Can you work these out from the model? Positions are in its coordinate system, mm. Face numbers are marked on the shaded views. A direction names the side the tool comes from. Round coordinates to 2 decimals unless told otherwise and drop trailing zeros. Order: outer loops, then holes, each group sorted by start corner. A loop starts at its lowest first (then second) coordinate and runs counter-clockwise, first axis right, second up. Notation, with made-up numbers: (10.25, -12) -> (64.25, -12) arc R29 ccw to (64.25, 13) -> close; hole circle Ø3 at (10.5, 52.25). An arc over 180 degrees is marked (long way). Use a Markdown table: item, result. Add a question column.
Q1. If we section it at A-A on y = 0: List the corners of the cut face in (x, z) for me, plus the area to 3 significant figures.
Q2. If we section it at D-D on z = 18.5: List the corners of the cut face in (x, y) for me, plus the area to 3 significant figures.
Q3. I'm going to push flat-ended pins straight in: pin 1 Ø3 at (x, y) = (25.5, -107) entering from -Z; pin 2 Ø2 at (x, z) = (23.5, 11) entering from +Y; pin 3 Ø6 at (x, y) = (16, 12) entering from +Z. Where does each tip first touch, or does it pass through?
Q4. If we section it at B-B on z = 0: List the corners of the cut face in (x, y) for me.
Q5. For the marked faces 1, 2 and 3, which set-ups out of +Z, -Z, +X, -X, +Y, -Y let a thin tool reach every point of the face, with its end or its side?
Q6. If we section it at C-C on y = -104.5: List the corners of the cut face in (x, z) for me.
Q7. I need wall thicknesses on line 1 along Y through (x, z) = (13, 43.5); line 2 along Y through (x, z) = (15.75, 35.5); line 3 along Z through (x, y) = (4.25, 44). Which ranges of each line are inside material? Lowest first, please. Write a range as [from, to].
Q8. We'd pull the mould along Y, two halves only. Please class the marked faces 4, 5, 6 and 7: +Y half, -Y half, draft (parallel to the pull), parting line (faces both ways), or undercut.
```python
from build123d import *

# Parameters (mm, degrees)
BASPROSKE_W              = 30
BASPROSKE_H              = 55
TOOTHCUT_DEPTH           = 84.366660003
TEETHCUTS_COUNT          = 20
BORSKE_R                 = 2.5
BORE_DEPTH               = 50.0000508
EXTRUDE_1_DEPTH          = 30
CUT_EXTRUDE_1_DEPTH      = 158.555338193
CUT_EXTRUDE_1_DEPTH_BACK = 158.555338193
SKETCH_7_R               = 2.5


with BuildPart() as part:
    # BasProSke → Base-Revolve (revolve)
    with BuildSketch(Plane(origin=(0, 0, 0), x_dir=(1, 0, 0), z_dir=(0, 1, 0)), mode=Mode.PRIVATE) as base_revolve_sk:
        with Locations((15, 27.5)):
            Rectangle(BASPROSKE_W, BASPROSKE_H)
    revolve(base_revolve_sk.sketch.rotate(Axis((-10, 0, 0), (1, 0, 0)), 180), axis=Axis((-10, 0, 0), (1, 0, 0)))

    # TooCutSke → ToothCut (cut, through all)
    with BuildSketch(Plane(origin=(0, 0, 0), x_dir=(0, 0, -1), z_dir=(1, 0, 0))):
        with BuildLine():
            ThreePointArc((2.464838288, 43.679509764), (0, 43.749), (-2.464838288, 43.679509764))
            ThreePointArc((-2.464838288, 43.679509764), (-4.057398861, 49.476814676), (-7.300899231, 54.538899105))
            ThreePointArc((-7.300899231, 54.538899105), (0, 55.0254), (7.300899231, 54.538899105))
            ThreePointArc((7.300899231, 54.538899105), (4.057398861, 49.476814676), (2.464838288, 43.679509764))
        make_face()
    toothcut = extrude(amount=TOOTHCUT_DEPTH, mode=Mode.SUBTRACT)

    # TeethCuts: ToothCut ×20 about axis
    teethcuts_axis = Axis((0, 0, 0), (1, 0, 0))
    for i in range(1, TEETHCUTS_COUNT):
        add(toothcut.rotate(teethcuts_axis, i * 360 / TEETHCUTS_COUNT), mode=Mode.SUBTRACT)

    # BorSke → Bore (cut, symmetric)
    with BuildSketch(Plane(origin=(0, 0, 0), x_dir=(0, 0, -1), z_dir=(1, 0, 0))):
        with Locations(Location((0, 0, 0), (0, 0, 180))):
            Circle(BORSKE_R)
    extrude(amount=BORE_DEPTH, both=True, mode=Mode.SUBTRACT)

    # 草图6 → 凸台-拉伸1 (add)
    with BuildSketch(Plane(origin=(30, 0, 0), x_dir=(0, 0, -1), z_dir=(1, 0, 0))):
        with BuildLine():
            Line((-4.466100318, -43.081201999), (11.177346186, -141.850036058))
            Line((11.177346186, -141.850036058), (33.20378387, -138.361391053))
            Line((33.20378387, -138.361391053), (17.560337366, -39.592556994))
            ThreePointArc((17.560337366, -39.592556994), (6.77314241, -42.763938152), (-4.466100318, -43.081201999))
        make_face()
    extrude(amount=-EXTRUDE_1_DEPTH)

    # 草图7 → 切除-拉伸1 (cut, two sides: drawn at the far end of the back side and taken through both)
    with BuildSketch(Plane(origin=(0, -1.744322502, 11.013218842), x_dir=(1, 0, 0), z_dir=(0, -0.15643446504023845, 0.9876883405951365)).offset(-CUT_EXTRUDE_1_DEPTH_BACK)):
        with Locations(Location((15, -130.568148899, 0), (0, 0, 270))):
            Circle(SKETCH_7_R)
    extrude(amount=CUT_EXTRUDE_1_DEPTH + CUT_EXTRUDE_1_DEPTH_BACK, mode=Mode.SUBTRACT)


solid = part.part
```
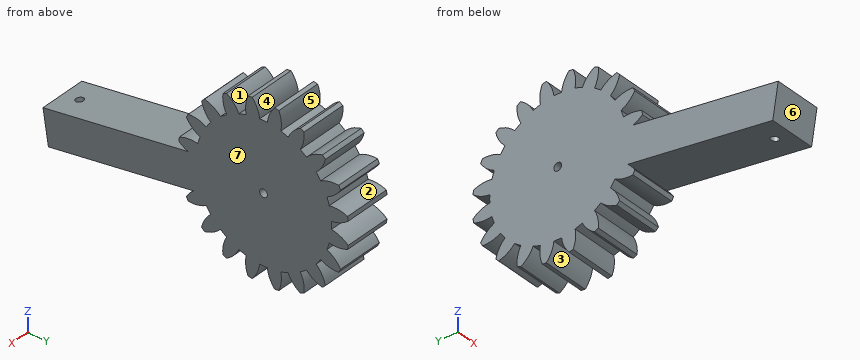
Answer below:
| question | item | result |
|---|---|---|
| 1 | outline | (0, -43.75) -> (30, -43.75) -> (30, -2.5) -> (0, -2.5) -> close; (0, 2.5) -> (30, 2.5) -> (30, 43.75) -> (0, 43.75) -> close |
| 1 | area | 2,470 mm² |
| 2 | outline | (0, -45.04) -> (30, -45.04) -> (30, 45.04) -> (0, 45.04) -> close |
| 2 | area | 2,700 mm² |
| 3 | pin 1 | z = -28.47 |
| 3 | pin 2 | y = 53.91 |
| 3 | pin 3 | z = 54.26 |
| 4 | outline | (0, -71.28) -> (30, -71.28) -> (30, -2.5) -> (0, -2.5) -> close; (0, 2.5) -> (30, 2.5) -> (30, 43.75) -> (0, 43.75) -> close |
| 5 | face 1 | +Z, +X, -X |
| 5 | face 2 | +X, -X |
| 5 | face 3 | -Z, +X, -X |
| 6 | outline | (0, -27.84) -> (30, -27.84) -> (30, -5.26) -> (0, -5.26) -> close |
| 7 | line 1 | [-26, -17.36], [-11.35, 11.35], [17.36, 26] |
| 7 | line 2 | [-39.11, -29.34], [-25.57, 25.57], [29.34, 39.11] |
| 7 | line 3 | [-26.07, -17.7], [-11.42, -2.51], [2.51, 11.42], [17.7, 26.07] |
| 8 | face 4 | undercut |
| 8 | face 5 | undercut |
| 8 | face 6 | -Y half |
| 8 | face 7 | draft |
